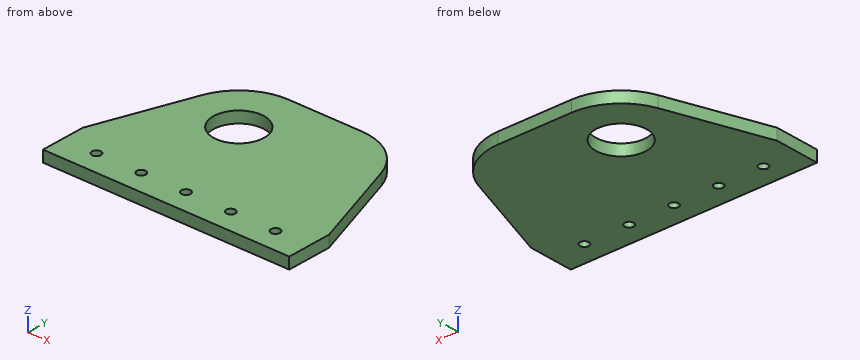
```python
from build123d import *

# Parameters (mm, degrees)
SKETCH1_R           = 14.2875
SKETCH1_R_2         = 2.54
BOSS_EXTRUDE1_DEPTH = 6.35


with BuildPart() as part:
    # Sketch1 → Boss-Extrude1 (new body)
    with BuildSketch(Plane.XY):
        with BuildLine():
            Line((49.043407506, 101.6), (90.656592494, 101.6))
            ThreePointArc((90.656592494, 101.6), (109.060504085, 95.721964327), (120.65, 80.264317364))
            Line((120.65, 80.264317364), (139.7, 25.4))
            Line((139.7, 25.4), (139.7, 0))
            Line((139.7, 0), (0, 0))
            Line((0, 0), (0, 25.4))
            Line((0, 25.4), (19.05, 80.264317364))
            ThreePointArc((19.05, 80.264317364), (30.639495915, 95.721964327), (49.043407506, 101.6))
        make_face()
        with Locations((49.043407506, 69.85)):
            Circle(SKETCH1_R, mode=Mode.SUBTRACT)
        with Locations((69.85, 12.7)):
            Circle(SKETCH1_R_2, mode=Mode.SUBTRACT)
        with Locations((95.25, 12.7)):
            Circle(SKETCH1_R_2, mode=Mode.SUBTRACT)
        with Locations((120.65, 12.7)):
            Circle(SKETCH1_R_2, mode=Mode.SUBTRACT)
        with Locations((44.45, 12.7)):
            Circle(SKETCH1_R_2, mode=Mode.SUBTRACT)
        with Locations((19.05, 12.7)):
            Circle(SKETCH1_R_2, mode=Mode.SUBTRACT)
    extrude(amount=BOSS_EXTRUDE1_DEPTH)


solid = part.part
```
Can you work these out from the model? Positions are in its coordinate system, mm. Coordinates: 2 decimals unless noted, no trailing zeros. Loops run counter-clockwise (first coordinate to the right, second up) from the corner with the lowest first, then second, coordinate; pieces in that order, holes last.
1) I need wall thicknesses on probe 1 along Y at (x, z) = (69.85, 3); probe 2 along X at (y, z) = (68.5, 5); probe 3 along X at (y, z) = (57, 6.25). Which ranges of each line are inside material? Lowest first, please.
2) Imagine slicing it at D-D on y = 82.5. List the corners of the cut face in (x, z) for me.
3) Imagine slicing it at A-A on y = 12.7. List the corners of the cut face in (x, z) for me.
4) For pin 1 (4.5 mm diameter, centred on x = 19.05, y = 12.7, fed in from -Z); pin 2 (1 mm diameter, centred on x = 105.5, z = 4.5, fed in from +Y), each with a flat end and sliding along its axis, tell me the tip position at first contact or that it passes through.
5) Imagine slicing it at C-C on x = 69.85. List the corners of the cut face in (y, z) for me.
6) Imagine slicing it at B-B on z = 2.75. State how many separate pieces and enclosed holes the cut face has, plus the area to 3 significant figures.
Completed:
1. probe 1: y = 0 to 10.16, 15.24 to 101.6
1. probe 2: x = 14.97 to 34.82, 63.27 to 124.73
1. probe 3: x = 10.97 to 42.8, 55.29 to 128.73
2. outline: (19.92, 0) - (42.4, 0) - (42.4, 6.35) - (19.92, 6.35) - close; (55.68, 0) - (119.78, 0) - (119.78, 6.35) - (55.68, 6.35) - close
3. outline: (0, 0) - (16.51, 0) - (16.51, 6.35) - (0, 6.35) - close; (21.59, 0) - (41.91, 0) - (41.91, 6.35) - (21.59, 6.35) - close; (46.99, 0) - (67.31, 0) - (67.31, 6.35) - (46.99, 6.35) - close; (72.39, 0) - (92.71, 0) - (92.71, 6.35) - (72.39, 6.35) - close; (97.79, 0) - (118.11, 0) - (118.11, 6.35) - (97.79, 6.35) - close; (123.19, 0) - (139.7, 0) - (139.7, 6.35) - (123.19, 6.35) - close
4. pin 1: passes through
4. pin 2: stops at y = 98.18
5. outline: (0, 0) - (10.16, 0) - (10.16, 6.35) - (0, 6.35) - close; (15.24, 0) - (101.6, 0) - (101.6, 6.35) - (15.24, 6.35) - close
6. separate pieces: 1
6. enclosed holes: 6
6. area: 11,200 mm2
